Job drawing, mm, ordinate dimensions from the low corner. One solid piece. A direction names the side the tool comes from. Coordinates: 2 decimals unless noted, no trailing zeros. Order: outer loops, then holes, each group sorted by start corner. A loop starts at its lowest first (then second) coordinate and runs counter-clockwise, first axis right, second up. Notation, with made-up numbers: M 53.25,32 L 59.25,32 A20 cw 59.25,58 Z; hole C 3,15.5 d11. An arc over 180 degrees is marked long. Write item = value, one per line.
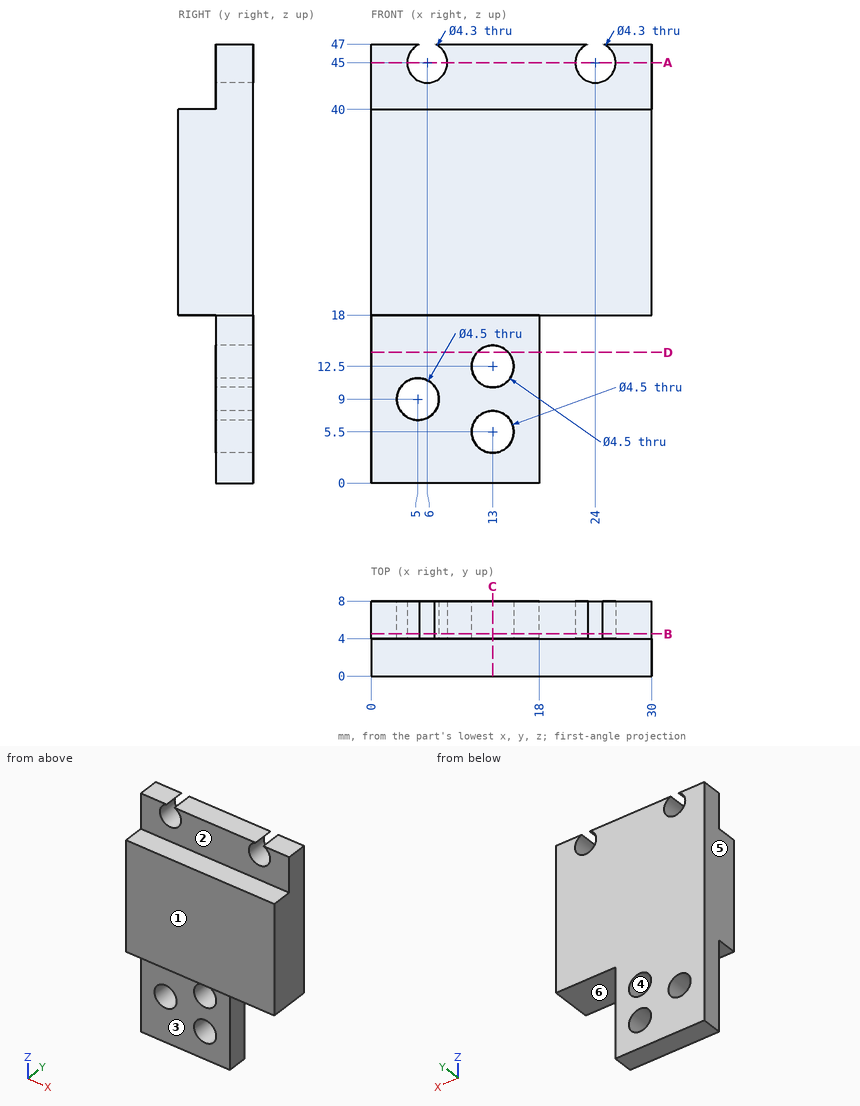
(1) Pull direction X, two halves, no side cores. Call the marked faces 4, 5 and 6: +X half, -X half, draft (parallel to the pull), parting line (faces both ways), or undercut.
Evaluation:
face_4 = undercut
face_5 = -X half
face_6 = draft
(2) Slice it at D-D, the plane z = 14. Write the cut outline in (x, y), then the cut area to 3 significant figures.
Evaluation:
outline = M 0,4 L 11.32,4 L 11.32,8 L 0,8 Z; M 14.68,4 L 18,4 L 18,8 L 14.68,8 Z
area = 58.6 mm²
(3) Slice it at B-B, the plane y = 4.5. Write the cut outline in (x, z).
Evaluation:
outline = M 0,0 L 18,0 L 18,18 L 30,18 L 30,47 L 24.79,47 A2.15 cw long 23.21,47 L 6.79,47 A2.15 cw long 5.21,47 L 0,47 Z; hole C 5,9 d4.5; hole C 13,5.5 d4.5; hole C 13,12.5 d4.5
(4) Pin check, flat tips, straight feed: pin 1 Ø2 at (x, y) = (9.5, 6) entering from -Z; pin 2 Ø2 at (x, y) = (4.5, 2) entering from -Z; pin 3 Ø4 at (x, z) = (24, 45) entering from +Y; pin 4 Ø6 at (x, z) = (5, 9) entering from -Y. Stop position of each tip, or through.
Evaluation:
pin_1 = 0
pin_2 = 18
pin_3 = through
pin_4 = 4
(5) Tool access for the marked faces 1, 2 and 3: list every direction of +Z, -Z, +X, -X, +Y, -Y with a clear straight run to the whole face (end or side of a thin tool).
Evaluation:
face_1 = +Z, -Z, +X, -X, -Y
face_2 = +Z, +X, -X, -Y
face_3 = -Z, +X, -X, -Y
(6) Slice it at A-A, the plane z = 45. Write the cut outline in (x, y).
Evaluation:
outline = M 0,4 L 3.85,4 L 3.85,8 L 0,8 Z; M 8.15,4 L 21.85,4 L 21.85,8 L 8.15,8 Z; M 26.15,4 L 30,4 L 30,8 L 26.15,8 Z
(7) Slice it at C-C, the plane x = 13. Write the cut outline in (y, z), then the cut area to 3 significant figures.
Evaluation:
outline = M 0,18 L 4,18 L 4,14.75 L 8,14.75 L 8,47 L 4,47 L 4,40 L 0,40 Z; M 4,0 L 8,0 L 8,3.25 L 4,3.25 Z; M 4,7.75 L 8,7.75 L 8,10.25 L 4,10.25 Z
area = 240 mm²
(8) Wall check: line 1 (Z direction, x = 13, y = 6.9); line 2 (X direction, y = 5.35, z = 12.5); line 3 (Z direction, x = 18.5, y = 7). Give the ranges that are in metal, low to high. Write a range as from..to.
Evaluation:
line_1 = 0..3.25, 7.75..10.25, 14.75..47
line_2 = 0..10.75, 15.25..18
line_3 = 18..47
